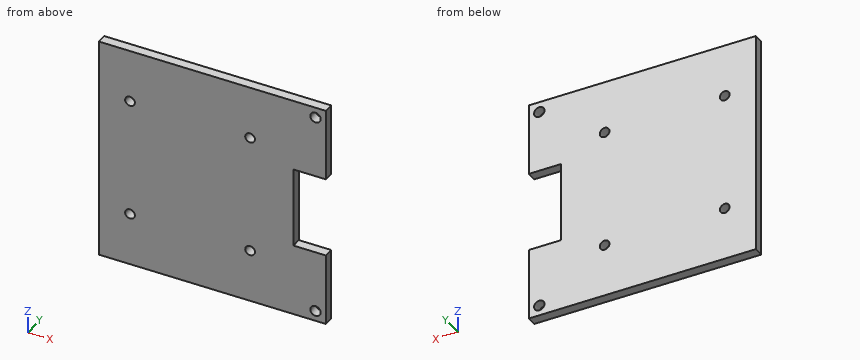
Autodesk Inventor part; units mm, degrees
ref_plane "YZ Plane" through (0, 0, 0) normal (1, 0, 0) x (0, 1, 0)
ref_plane "XZ Plane" through (0, 0, 0) normal (0, 1, 0) x (-1, 0, 0)
ref_plane "XY Plane" through (0, 0, 0) normal (0, 0, 1) x (1, 0, 0)
sketch "Эскиз1" plane through (0, 0, 0) normal (0, 1, 0) x (-1, 0, 0)
  line L0 (-35, 35) -> (35, 35)
  line L1 (35, 35) -> (35, -35)
  line L2 (35, -35) -> (-35, -35)
  line L3 (-35, -35) -> (-35, 35)
  line L4 (-35, 35) -> (35, -35) construction
  line L5 (35, 35) -> (-35, -35) construction
  line L6 (-35, 35) -> (-31.7678, 31.7678)
  circle A0 centre (-31.7678, 31.7678) radius 1.6
  line L7 (-35, -35) -> (-31.7678, -31.7678)
  circle A1 centre (-31.7678, -31.7678) radius 1.6
  point P0 (0, 0)
  dimension "d0" = 70
  dimension "d1" = 70
  dimension "d2" = 4.571
  dimension "d3" = 3.2
  dimension "d4" = 4.571
  dimension "d5" = 3.2
extrude "Выдавливание1" add sketch "Эскиз1" along normal blind 3
sketch "Эскиз2" plane through (35, 0, 35) normal (1, 0, 0) x (0, 0, -1)
  line L0 (35, 0) -> (35, 3)
  line L1 (0, 3) -> (70, 3)
  line L2 (22.5, 0) -> (47.5, 0)
  line L3 (47.5, 0) -> (47.5, 3)
  line L4 (47.5, 3) -> (22.5, 3)
  line L5 (22.5, 3) -> (22.5, 0)
  line L6 (22.5, 0) -> (47.5, 3) construction
  line L7 (47.5, 0) -> (22.5, 3) construction
  point P0 (35, 1.5)
  dimension "d8" = 25
extrude "Выдавливание2" cut sketch "Эскиз2" against normal blind 10
sketch "Эскиз3" plane through (0, 3, 0) normal (0, 1, 0) x (1, 0, 0)
  line L0 (-28.375, -21.875) -> (-28.375, 21.875)
  line L1 (14.625, -21.875) -> (-28.375, -21.875)
  line L2 (14.625, 21.875) -> (14.625, -21.875)
  line L3 (-28.375, 21.875) -> (14.625, 21.875)
  circle A0 centre (11.625, -18.5) radius 1.5
  circle A1 centre (-25.375, -18.5) radius 1.5
  circle A2 centre (-25.375, 18.5) radius 1.5
  circle A3 centre (11.625, 18.5) radius 1.5
  point P0 (0, 0)
  point P1 (-6.875, 0)
extrude "Выдавливание3" cut sketch "Эскиз3" against normal blind 10 contours A0 | A1 | A2 | A3
equation "\"d4\" = d2"
equation "\"d5\" = d3"
properties part number "000.107 - Правая стенка среднего сегмента"
For this review, take the finished solid that the model builds, in its own axes (mm). Give positions to 0.01 mm unless a question says otherwise; leave off trailing zeros. Loops run counter-clockwise (first coordinate to the right, second up) from the corner with the lowest first, then second, coordinate; pieces in that order, holes last. Notation, with made-up numbers: M 43.5,72.25 L 54.5,72.25 A29 cw 54.5,101.25 Z; hole C -31,-19.5 d1. An arc over 180 degrees is marked long. One line per item, written item: value. Start each with the question number.
Q1. For L1, parallel to X at y = 0.65, z = 18.5 (3 decimals); L2, parallel to Z at x = 13, y = 0.3; L3, parallel to Z at x = 27.5, y = 1.7, list the stretches that pass through material, from the lowest coordinate up.
Q2. Add section C-C (y = 2.55). Give the boundary of the cut face in (x, z) (3 decimals).
Q3. Add section B-B (x = 27.5). Give the boundary of the cut face in (y, z), and give its area (3 significant figures).
Q4. Add section D-D (z = 7). Give the boundary of the cut face in (x, y), and give its area (3 significant figures).
Q5. Clearance check with flat-ended pins moving along their axes: pin 1 Ø5 at (x, z) = (11.625, -18.5) entering from -Y; pin 2 Ø2.5 at (x, z) = (31.77, -31.77) entering from +Y. State where each tip first meets the part, or that it passes through.
Q6. Add section A-A (z = 18.5). Give the boundary of the cut face in (x, y) (3 decimals).
Reply:
1. L1: -35 to -26.875, -23.875 to 10.125, 13.125 to 35
1. L2: -35 to -19.1, -17.9 to 17.9, 19.1 to 35
1. L3: -35 to -12.5, 12.5 to 35
2. outline: M -35,-35 L 35,-35 L 35,-12.5 L 25,-12.5 L 25,12.5 L 35,12.5 L 35,35 L -35,35 Z; hole C -25.375,-18.5 d3; hole C -25.375,18.5 d3; hole C 11.625,-18.5 d3; hole C 11.625,18.5 d3; hole C 31.768,-31.768 d3.2; hole C 31.768,31.768 d3.2
3. outline: M 0,-35 L 3,-35 L 3,-12.5 L 0,-12.5 Z; M 0,12.5 L 3,12.5 L 3,35 L 0,35 Z
3. area: 135 mm²
4. outline: M -35,0 L 25,0 L 25,3 L -35,3 Z
4. area: 180 mm²
5. pin 1: y = 0
5. pin 2: through
6. outline: M -35,0 L -26.875,0 L -26.875,3 L -35,3 Z; M -23.875,0 L 10.125,0 L 10.125,3 L -23.875,3 Z; M 13.125,0 L 35,0 L 35,3 L 13.125,3 Z
